CAD build for the part. Positions are in the model's coordinates, mm. Round coordinates to 2 decimals unless told otherwise and drop trailing zeros. Write each loop counter-clockwise with the first axis right and the second up, starting at its lowest first coordinate (ties: lowest second). Pieces come first, ordered by that corner, then holes. Notation, with made-up numbers: (-28, 80.5) -> (25, 80.5) arc R8 ccw to (25, 93.5) -> close; hole circle Ø5 at (32.5, 1). An arc over 180 degrees is marked (long way). Answer in a Markdown table with one row per item. Add a question column.
```python
from build123d import *

# Parameters (mm, degrees)
F0_R     = 1.524
F0_R_2   = 10.75
F0_R_3   = 16.1
F1_DEPTH = 2


with BuildPart() as f1:
    # F0 (on Front) → F1 (new body)
    with BuildSketch(Plane.XZ):
        with BuildLine():
            Line((-24.75, 6), (-24.75, 0))
            Line((-24.75, 0), (-24.75, -6))
            ThreePointArc((-24.75, -6), (-19.477922, -18.727922), (-6.75, -24))
            Line((-6.75, -24), (70.1, -24))
            ThreePointArc((70.1, -24), (80.706602, -19.606602), (85.1, -9))
            Line((85.1, -9), (85.1, 0))
            Line((85.1, 0), (85.1, 9))
            ThreePointArc((85.1, 9), (80.706602, 19.606602), (70.1, 24))
            Line((70.1, 24), (-6.75, 24))
            ThreePointArc((-6.75, 24), (-19.477922, 18.727922), (-24.75, 6))
        make_face()
        with Locations((-11.5062, -11.5062)):
            Circle(F0_R, mode=Mode.SUBTRACT)
        with Locations((11.5062, -11.5062)):
            Circle(F0_R, mode=Mode.SUBTRACT)
        with Locations((37.3188, -14.6812)):
            Circle(F0_R, mode=Mode.SUBTRACT)
        with Locations((66.6812, -14.6812)):
            Circle(F0_R, mode=Mode.SUBTRACT)
        Circle(F0_R_2, mode=Mode.SUBTRACT)
        with Locations((-11.5062, 11.5062)):
            Circle(F0_R, mode=Mode.SUBTRACT)
        with Locations((11.5062, 11.5062)):
            Circle(F0_R, mode=Mode.SUBTRACT)
        with Locations((52, 0)):
            Circle(F0_R_3, mode=Mode.SUBTRACT)
        with Locations((37.3188, 14.6812)):
            Circle(F0_R, mode=Mode.SUBTRACT)
        with Locations((66.6812, 14.6812)):
            Circle(F0_R, mode=Mode.SUBTRACT)
    extrude(amount=F1_DEPTH)


solid = f1.part
```
Item 1: Drill centre lines: probe 1 along Z at (x, y) = (38.5, -0.65); probe 2 along X at (y, z) = (-1.3, 12); probe 3 along X at (y, z) = (-0.7, -1). Where is each one in solid material? Low to high.
Item 2: Pin check, flat tip, straight feed: pin 1 (13 mm diameter, centred on x = 0, z = 0, fed in from -Y). Stop position of the tip, or through.
Item 3: Saw through at A-A on x = 52. Give the cut face in (y, z), then the cut area to 3 significant figures.
Item 4: Saw through at C-C on x = 0. Give the cut face in (y, z).
Item 5: Two-plate mould, pull along Z, no slides. Class faces 1 (the flat face through (31, -1, -24)), 2 (the cylindrical face through (68.09, -0.99, -15.26)), 3 (the flat face through (32, -1, 24)): +Z half, -Z half, draft (parallel to the pull), parting line (faces both ways), or undercut.
Item 6: Saw through at B-B on z = 3.5. Give the cut face in (x, y).
Item 7: Saw through at D-D on y = -1.35. Count the separate pieces of the cut face and the enclosed holes in it, then the cut area to 3 significant figures.
Recorded:
| question | item | result |
|---|---|---|
| 1 | probe 1 | -24 to -15.64, -13.72 to -8.77, 8.77 to 13.72, 15.64 to 24 |
| 1 | probe 2 | -23.72 to -12.95, -10.06 to 10.06, 12.95 to 41.27, 62.73 to 84.8 |
| 1 | probe 3 | -24.75 to -10.7, 10.7 to 35.93, 68.07 to 85.1 |
| 2 | pin 1 | through |
| 3 | outline | (-2, -24) -> (0, -24) -> (0, -16.1) -> (-2, -16.1) -> close; (-2, 16.1) -> (0, 16.1) -> (0, 24) -> (-2, 24) -> close |
| 3 | area | 31.6 mm2 |
| 4 | outline | (-2, -24) -> (0, -24) -> (0, -10.75) -> (-2, -10.75) -> close; (-2, 10.75) -> (0, 10.75) -> (0, 24) -> (-2, 24) -> close |
| 5 | face 1 | -Z half |
| 5 | face 2 | undercut |
| 5 | face 3 | +Z half |
| 6 | outline | (-24.75, -2) -> (-10.16, -2) -> (-10.16, 0) -> (-24.75, 0) -> close; (10.16, -2) -> (36.29, -2) -> (36.29, 0) -> (10.16, 0) -> close; (67.71, -2) -> (85.1, -2) -> (85.1, 0) -> (67.71, 0) -> close |
| 7 | separate pieces | 1 |
| 7 | enclosed holes | 10 |
| 7 | area | 3,800 mm2 |
